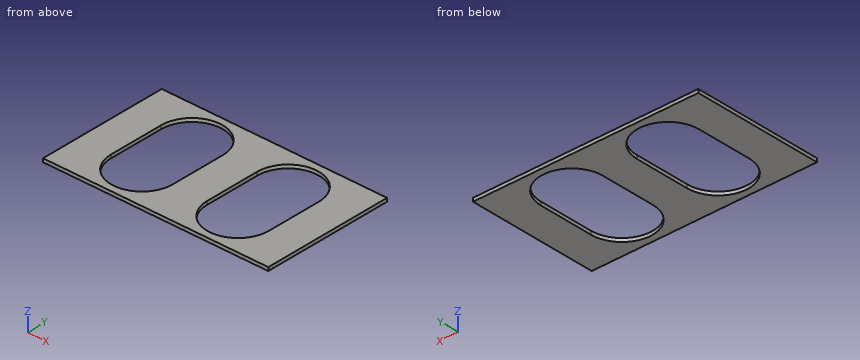
from build123d import *

# Parameters (mm, degrees)
SKETCH_1_W      = 328
SKETCH_1_H      = 190
EXTRUDE_1_DEPTH = 5


with BuildPart() as part:
    # Эскиз1 → Бобышка-Вытянуть1 (new body)
    with BuildSketch(Plane.XY):
        Rectangle(SKETCH_1_W, SKETCH_1_H)
        with BuildLine():
            Line((-25, 40), (-25, -40))
            ThreePointArc((-25, -40), (-70, -85), (-115, -40))
            Line((-115, -40), (-115, 40))
            ThreePointArc((-115, 40), (-70, 85), (-25, 40))
        make_face(mode=Mode.SUBTRACT)
        with BuildLine():
            Line((25, 40), (25, -40))
            ThreePointArc((25, -40), (70, -85), (115, -40))
            Line((115, -40), (115, 40))
            ThreePointArc((115, 40), (70, 85), (25, 40))
        make_face(mode=Mode.SUBTRACT)
    extrude(amount=EXTRUDE_1_DEPTH)


solid = part.part
Geometry: final body of the model. Coordinates: model frame, mm. Round coordinates to 2 decimals unless told otherwise and drop trailing zeros. Loops run counter-clockwise (first coordinate to the right, second up) from the corner with the lowest first, then second, coordinate; pieces in that order, holes last.
Q1. Section B-B on x = -70. Return loops of the section in (y, z), plus the area to 3 significant figures.
Q2. Section D-D on y = -67. Return loops of the section in (x, z), plus the area to 3 significant figures.
Q3. Material intervals for L1, parallel to X at y = 21, z = 0.9; L2, parallel to X at y = -66, z = 2.3; L3, parallel to Y at x = 43.5, z = 0.95, sorted ascending.
Q4. Section C-C on z = 3.55. Return loops of the section in (x, y), plus the area to 3 significant figures.
Q5. Section A-A on y = -19.5. Return loops of the section in (x, z).
Evaluation:
1. outline: (-95, 0) - (-85, 0) - (-85, 5) - (-95, 5) - close; (85, 0) - (95, 0) - (95, 5) - (85, 5) - close
1. area: 100 mm2
2. outline: (-164, 0) - (-106, 0) - (-106, 5) - (-164, 5) - close; (-34, 0) - (34, 0) - (34, 5) - (-34, 5) - close; (106, 0) - (164, 0) - (164, 5) - (106, 5) - close
2. area: 920 mm2
3. L1: x = -164 to -115, -25 to 25, 115 to 164
3. L2: x = -164 to -106.73, -33.27 to 33.27, 106.73 to 164
3. L3: y = -95 to -76.37, 76.37 to 95
4. outline: (-164, -95) - (164, -95) - (164, 95) - (-164, 95) - close; hole (-115, -40) arc R45 ccw to (-25, -40) - (-25, 40) arc R45 ccw to (-115, 40) - close; hole (25, -40) arc R45 ccw to (115, -40) - (115, 40) arc R45 ccw to (25, 40) - close
4. area: 35,200 mm2
5. outline: (-164, 0) - (-115, 0) - (-115, 5) - (-164, 5) - close; (-25, 0) - (25, 0) - (25, 5) - (-25, 5) - close; (115, 0) - (164, 0) - (164, 5) - (115, 5) - close
